from build123d import *

# Parameters (mm, degrees)
SKETCH2_W           = 12.7
SKETCH2_H           = 15.4
BOSS_EXTRUDE1_DEPTH = 3.15
SKETCH3_W           = 0.5
SKETCH3_H           = 3
BOSS_EXTRUDE2_DEPTH = 7
SKETCH4_R           = 0.4
CUT_EXTRUDE1_DEPTH  = 23.225
CHAMFER1_SIZE       = 0.7
BOSS_EXTRUDE3_DEPTH = 3
FILLET1_R           = 0.5


with BuildPart() as part:
    # Sketch1 → Revolve1 (revolve)
    with BuildSketch(Plane.XY):
        with BuildLine():
            Line((0, 0), (0, 12.35))
            Line((0, 12.35), (3.5, 12.35))
            ThreePointArc((3.5, 12.35), (4.678895206, 15.196104794), (7.525, 16.375))
            Line((7.525, 16.375), (7.525, 14.95))
            Line((7.525, 14.95), (20, 14.95))
            Line((20, 14.95), (20, 12.5))
            Line((20, 12.5), (16.75, 12.5))
            Line((16.75, 12.5), (16.75, 0))
            Line((16.75, 0), (0, 0))
        make_face()
    revolve(axis=Axis((16.75, 0, 0), (-1, 0, 0)))

    # Sketch2 → Boss-Extrude1 (add)
    with BuildSketch(Plane(origin=(16.75, 0, 0), x_dir=(0, 0, -1), z_dir=(1, 0, 0))):
        Rectangle(SKETCH2_W, SKETCH2_H)
    extrude(amount=BOSS_EXTRUDE1_DEPTH)

    # Sketch3 → Boss-Extrude2 (add)
    with BuildSketch(Plane(origin=(19.9, 0, 0), x_dir=(0, 0, -1), z_dir=(1, 0, 0))):
        with Locations((5.6, 3.4)):
            Rectangle(SKETCH3_W, SKETCH3_H)
        with Locations((5.6, -3.4)):
            Rectangle(SKETCH3_W, SKETCH3_H)
    extrude(amount=BOSS_EXTRUDE2_DEPTH)

    # Sketch4 → Cut-Extrude1 (cut, through all)
    with BuildSketch(Plane(origin=(0, 0, -5.85), x_dir=(-1, 0, 0), z_dir=(0, 0, -1))):
        with Locations((-24.75, 3.4)):
            Circle(SKETCH4_R)
        with Locations((-24.75, -3.4)):
            Circle(SKETCH4_R)
    extrude(amount=-CUT_EXTRUDE1_DEPTH, mode=Mode.SUBTRACT)

    # Chamfer1
    chamfer1_edges = [part.edges().sort_by_distance(p)[0] for p in [
        (26.9, 1.9, -5.6),
        (26.9, 4.9, -5.6),
        (26.9, -4.9, -5.6),
        (26.9, -1.9, -5.6),
    ]]
    chamfer(chamfer1_edges, length=CHAMFER1_SIZE)

    # Sketch5 → Boss-Extrude3 (add, symmetric)
    with BuildSketch(Plane(origin=(0, 0, 0), x_dir=(1, 0, 0), z_dir=(0, 1, 0))):
        Polygon((17.666687605, -14.95), (10.525, -17.45), (8.866687605, -14.95), (8.866687605, -13.95), (17.666687605, -13.95), align=None)
        Polygon((8.866687605, 13.95), (8.866687605, 14.95), (10.525, 17.45), (17.666687605, 14.95), (17.666687605, 13.95), align=None)
    extrude(amount=BOSS_EXTRUDE3_DEPTH, both=True)

    # Fillet1
    fillet1_edges = [part.edges().sort_by_distance(p)[0] for p in [
        (0, -12.35, 0),
    ]]
    fillet(fillet1_edges, radius=FILLET1_R)


solid = part.part
Could you check a few things on this model? Use its own coordinates, in mm. A direction names the side the tool comes from. Give positions to 0.01 mm unless a question says otherwise; leave off trailing zeros. Loops run counter-clockwise (first coordinate to the right, second up) from the corner with the lowest first, then second, coordinate; pieces in that order, holes last. Notation, with made-up numbers: (-10, 3) -> (29, 3) arc R29 cw to (29, 28) -> close; hole circle Ø8 at (8, 70.5). An arc over 180 degrees is marked (long way). Answer as CSV lines item,"result". Start each with the question number.
(1) If we section it at A-A on z = 0: Write out the boundary of the cut face in (x, y) (3 decimals).
(2) We'd pull the mould along Y, two halves only. Please class faces 1 (the flat face through (18, 0, -6.35)), 2 (the cylindrical face through (13.85, -3.241, 14.594)), 3 (the flat face through (12, 3, 16)): released by +Y, released by -Y, zero draft, split by the parting line, or undercut.
(3) Which directions (+Z, -Z, +X, -X, +Y, -Y) give clear straight access to the entire face, cutting with the end or side of a thin tool? Please do faces 4 (the cylindrical face through (2.02, 11.78, -3.71)), 5 (the flat face through (9.71, -0.04, 16.22)), 6 (the flat face through (18, 7.7, 0)).
(4) I need wall thicknesses on probe 1 along Z at (x, y) = (17.85, 0); probe 2 along Y at (x, z) = (24.75, -5.5); probe 3 along Z at (x, y) = (18.5, -3.5). Which ranges of each line are inside material? Lowest first, please.
(5) I'm going to push flat-ended pins straight in: pin 1 Ø12 at (y, z) = (8, 0.5) entering from +X; pin 2 Ø2.5 at (x, z) = (18.5, -3) entering from +Y; pin 3 Ø1.5 at (x, y) = (24, -3) entering from +Z. Where does each tip first touch, or does it pass through?
Computed:
1,outline,"(0, -11.85) arc R0.5 ccw to (0.5, -12.35) -> (3.5, -12.35) arc R4.025 ccw to (7.525, -16.375) -> (7.525, -14.95) -> (20, -14.95) -> (20, -12.5) -> (16.75, -12.5) -> (16.75, -7.7) -> (19.9, -7.7) -> (19.9, 7.7) -> (16.75, 7.7) -> (16.75, 12.5) -> (20, 12.5) -> (20, 14.95) -> (7.525, 14.95) -> (7.525, 16.375) arc R4.025 ccw to (3.5, 12.35) -> (0.5, 12.35) arc R0.5 ccw to (0, 11.85) -> close"
2,face 1,"undercut"
2,face 2,"split by the parting line"
2,face 3,"released by +Y"
3,face 4,"-X"
3,face 5,"+Z, +Y, -Y"
3,face 6,"+X"
4,probe 1,"z = -14.95 to -12.5, -6.35 to 6.35, 12.5 to 14.95"
4,probe 2,"y = -4.9 to -3.8, -3 to -1.9, 1.9 to 3, 3.8 to 4.9"
4,probe 3,"z = -14.53 to -12, -6.35 to 6.35, 12 to 14.53"
5,pin 1,"stops at x = 20"
5,pin 2,"stops at y = 14.85"
5,pin 3,"stops at z = -5.35"
